Source: CAD feature listing. Evaluate the final solid. Frame: model axes, mm. Face numbers are marked on the shaded views. A direction names the side the tool comes from. Coordinates: 2 decimals unless noted, no trailing zeros. Loops run counter-clockwise (first coordinate to the right, second up) from the corner with the lowest first, then second, coordinate; pieces in that order, holes last. Notation, with made-up numbers: M -17,-1 L 10,-1 A23 cw 10,14 Z; hole C 61,60 d4. An arc over 180 degrees is marked long. One line per question, with ' | ' between items. Start each with the question number.
1. Section query A-A, the plane y = 960. Output: boundary loops of the cut face in (x, z).
2. Pin query (flat end, axial travel): P1, Ø9, axis at x = -104, z = 54.5, coming from the +Y side; P2, Ø1.5, axis at y = 285.5, z = 47.5, coming from the +X side; P3, Ø18, axis at x = 144, z = 43.5, coming from the -Y side. Return the tip coordinate at first contact, or that it passes through.
3. Section query B-B, the plane y = 95. Output: boundary loops of the cut face in (x, z).
4. Ray query, probe 1 along X at (y, z) = (525, 49); probe 2 along X at (y, z) = (960, 52); probe 3 along X at (y, z) = (670, 54). Return the intervals inside material, ascending.
5. Section query C-C, the plane z = 44.5. State how many separate pieces and enclosed holes the cut face has, and give its area (3 significant figures).
6. Section query D-D, the plane y = 611. Output: boundary loops of the cut face in (x, z).
7. Access query for the marked faces 1, 2, 3, 4 and 5. Directions: +Z, -Z, +X, -X, +Y, -Y. A direction counts if a zero-diameter tool reaches every point of the face in a straight line with its end or side. Return the directions, or none.
8. Mould query, pull axis X, two halves, no side actions, for the marked faces 6, 7, 8 and 9. Classes: pulls with the +X half, pulls with the -X half, needs draft (parallel to the pull), parting line crosses it, or undercut.
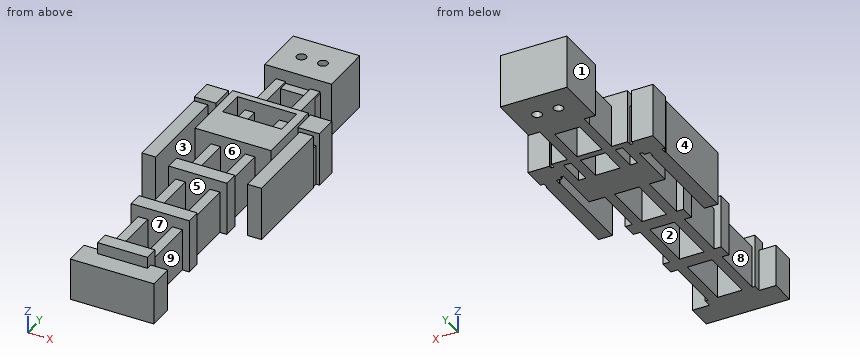
```python
from build123d import *

# Parameters (mm, degrees)
SKETCH1_W             = 218
SKETCH1_H             = 66
BOSS_EXTRUDE1_DEPTH   = 110
SKETCH1_W_2           = 25.4
SKETCH1_H_2           = 820
BOSS_EXTRUDE1_2_DEPTH = 110
BOSS_EXTRUDE1_3_DEPTH = 110
SKETCH2_W             = 130
SKETCH2_H             = 36
SKETCH2_W_2           = 152
SKETCH2_H_2           = 38
SKETCH2_W_3           = 198
SKETCH2_H_3           = 180
SKETCH2_W_4           = 154
SKETCH2_H_4           = 72
SKETCH2_W_5           = 56
SKETCH2_H_5           = 60
SKETCH2_W_6           = 36
SKETCH2_H_6           = 250
SKETCH2_W_7           = 174
SKETCH2_H_7           = 136
SKETCH2_R             = 12.5
BOSS_EXTRUDE2_DEPTH   = 140
SKETCH3_W             = 24
SKETCH3_H             = 44
SKETCH3_W_2           = 32
SKETCH3_H_2           = 30
SKETCH3_W_3           = 116
SKETCH3_H_3           = 36
BOSS_EXTRUDE3_DEPTH   = 105


with BuildPart() as part:
    # Sketch1 → Boss-Extrude1 (new body)
    with BuildSketch(Plane.XY):
        with Locations((0, 33)):
            Rectangle(SKETCH1_W, SKETCH1_H)
    extrude(amount=BOSS_EXTRUDE1_DEPTH)



with BuildPart() as body_2:
    # Sketch1 → Boss-Extrude1 2 (new body)
    with BuildSketch(Plane.XY):
        with Locations((-45, 485)):
            Rectangle(SKETCH1_W_2, SKETCH1_H_2)
    extrude(amount=BOSS_EXTRUDE1_2_DEPTH)


with BuildPart() as body_3:
    # Sketch1 → Boss-Extrude1 3 (new body)
    with BuildSketch(Plane.XY):
        with Locations((45, 485)):
            Rectangle(SKETCH1_W_2, SKETCH1_H_2)
    extrude(amount=BOSS_EXTRUDE1_3_DEPTH)


with BuildPart() as part_1:
    add(part.part)

    add(body_2.part)  # Boss-Extrude2 merges body 2

    add(body_3.part)  # Boss-Extrude2 merges body 3
    # Sketch2 → Boss-Extrude2 (add)
    # profile 1 of 9: a face of its own
    with BuildSketch(Plane.XY):
        with Locations((0, 68)):
            Rectangle(SKETCH2_W, SKETCH2_H)
    # profile 2 of 9: a face of its own
    with BuildSketch(Plane.XY):
        with Locations((0, 250)):
            Rectangle(SKETCH2_W_2, SKETCH2_H_2)
    # profile 3 of 9: a face of its own
    with BuildSketch(Plane.XY):
        with Locations((0, 430)):
            Rectangle(SKETCH2_W_2, SKETCH2_H_2)
    # profile 4 of 9: a face of its own
    with BuildSketch(Plane.XY):
        with Locations((0, 670)):
            Rectangle(SKETCH2_W_3, SKETCH2_H_3)
        with Locations((0, 707)):
            Rectangle(SKETCH2_W_4, SKETCH2_H_4, mode=Mode.SUBTRACT)
    # profile 5 of 9: a face of its own
    with BuildSketch(Plane.XY):
        with Locations((-135, 725)):
            Rectangle(SKETCH2_W_5, SKETCH2_H_5)
    # profile 6 of 9: a face of its own
    with BuildSketch(Plane.XY):
        with Locations((135, 725)):
            Rectangle(SKETCH2_W_5, SKETCH2_H_5)
    # profile 7 of 9: a face of its own
    with BuildSketch(Plane.XY):
        with Locations((-138, 555)):
            Rectangle(SKETCH2_W_6, SKETCH2_H_6)
    # profile 8 of 9: a face of its own
    with BuildSketch(Plane.XY):
        with Locations((138, 555)):
            Rectangle(SKETCH2_W_6, SKETCH2_H_6)
    # profile 9 of 9: a face of its own
    with BuildSketch(Plane.XY):
        with Locations((0, 960)):
            Rectangle(SKETCH2_W_7, SKETCH2_H_7)
        with Locations((-28, 960)):
            Circle(SKETCH2_R, mode=Mode.SUBTRACT)
        with Locations((28, 960)):
            Circle(SKETCH2_R, mode=Mode.SUBTRACT)
    extrude(amount=BOSS_EXTRUDE2_DEPTH)

    # Sketch3 → Boss-Extrude3 (add)
    with BuildSketch(Plane.XY):
        with Locations((-103, 725)):
            Rectangle(SKETCH3_W, SKETCH3_H)
        with Locations((103, 725)):
            Rectangle(SKETCH3_W, SKETCH3_H)
        with Locations((-138, 688)):
            Rectangle(SKETCH3_W_2, SKETCH3_H_2)
        with Locations((138, 688)):
            Rectangle(SKETCH3_W_2, SKETCH3_H_2)
        with Locations((0, 885)):
            Rectangle(SKETCH3_W_3, SKETCH3_H_3)
    extrude(amount=BOSS_EXTRUDE3_DEPTH)


solid = part_1.part
```
Taken from the geometry:
1) outline: M -87,0 L -40.5,0 L -40.5,140 L -87,140 Z; M -15.5,0 L 15.5,0 L 15.5,140 L -15.5,140 Z; M 40.5,0 L 87,0 L 87,140 L 40.5,140 Z
2) P1: y = 755 | P2: x = 57.7 | P3: y = 430
3) outline: M -57.7,0 L -32.3,0 L -32.3,110 L -57.7,110 Z; M 32.3,0 L 57.7,0 L 57.7,110 L 32.3,110 Z
4) probe 1: -156 to -120, -57.7 to -32.3, 32.3 to 57.7, 120 to 156 | probe 2: -87 to -40.5, -15.5 to 15.5, 40.5 to 87 | probe 3: -156 to -120, -99 to 99, 120 to 156
5) separate pieces: 1 | enclosed holes: 9 | area: 135,000 mm^2
6) outline: M -156,0 L -120,0 L -120,140 L -156,140 Z; M -99,0 L 99,0 L 99,140 L -99,140 Z; M 120,0 L 156,0 L 156,140 L 120,140 Z
7) face 1: +Z, -Z, -X, +Y | face 2: +Z, -Z | face 3: +Z, -Z, -Y | face 4: +Z, -Z, -X, -Y | face 5: +Z
8) face 6: undercut | face 7: undercut | face 8: pulls with the -X half | face 9: pulls with the +X half
